Autodesk Fusion 360 part; units mm, degrees
sketch "Sketch1" plane through (0, 0, 0) normal (0, 0, 1) x (1, 0, 0)
  line L0 (13, 7.5056) -> (0, 15.0111)
  line L1 (0, 15.0111) -> (-13, 7.5056)
  line L2 (-13, 7.5056) -> (-13, -7.5056)
  line L3 (-13, -7.5056) -> (0, -15.0111)
  line L4 (0, -15.0111) -> (13, -7.5056)
  line L5 (13, -7.5056) -> (13, 7.5056)
  dimension "d1" = 13
extrude "Extrude1" add sketch "Sketch1" along normal blind 1.5
sketch "Sketch2" plane through (0, 0, 1.5) normal (0, 0, 1) x (-1, 0, 0)
  line L0 (-13, 7.5056) -> (-13, -7.5056)
  line L1 (-13, -7.5056) -> (0, -15.0111)
  line L2 (0, -15.0111) -> (13, -7.5056)
  line L3 (13, -7.5056) -> (13, 7.5056)
  line L4 (13, 7.5056) -> (0, 15.0111)
  line L5 (0, 15.0111) -> (-13, 7.5056)
  circle A0 centre (0, 0) radius 3.1
  dimension "d4" = 6.2
extrude "Extrude2" cut sketch "Sketch2" against normal blind 13 contours A0
chamfer "Chamfer1" distance 0.75 angle 45 1 edges at (2.8902, -1.121, 1.5)
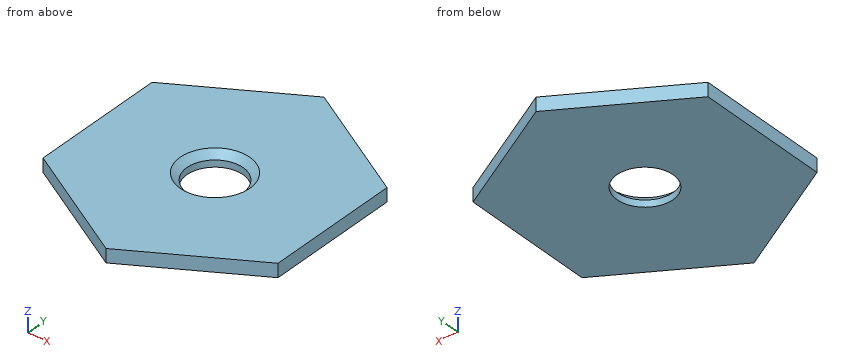
The model under review builds one solid part; all positions refer to its coordinate system, in mm. Round coordinates to 2 decimals unless told otherwise and drop trailing zeros. Order: outer loops, then holes, each group sorted by start corner. A loop starts at its lowest first (then second) coordinate and runs counter-clockwise, first axis right, second up.
(1) Take a section at A-A, the plane y = 0. State the section outline as (x, z) points.
Working result:
outline: (-13, 0) - (-3.1, 0) - (-3.1, 0.75) - (-3.85, 1.5) - (-13, 1.5) - close; (3.1, 0) - (13, 0) - (13, 1.5) - (3.85, 1.5) - (3.1, 0.75) - close
(2) Take a section at C-C, the plane y = -8. State the section outline as (x, z) points, plus the area to 3 significant figures.
Working result:
outline: (-12.14, 0) - (12.14, 0) - (12.14, 1.5) - (-12.14, 1.5) - close
area: 36.4 mm2
(3) Take a section at B-B, the plane x = 5.25. State the section outline as (y, z) points.
Working result:
outline: (-11.98, 0) - (11.98, 0) - (11.98, 1.5) - (-11.98, 1.5) - close
(4) For P1, Ø7, axis at x = 0, y = 0, coming from the -Z side, flat-tipped, find the tip position at first contact; note if it passes through.
Working result:
P1: stops at z = 0
(5) Wall thickness on L1, parallel to X at y = 0, z = 0.45; L2, parallel to X at y = -0.5, z = 1; L3, parallel to Y at x = 3, z = 1.45: over which ranges is each line inside the solid? List them lowest first.
Working result:
L1: x = -13 to -3.1, 3.1 to 13
L2: x = -13 to -3.31, 3.31 to 13
L3: y = -13.28 to -2.33, 2.33 to 13.28
